from build123d import *

# Parameters (mm, degrees)
SKETCH_1_R          = 25
SKETCH_1_R_2        = 15
EXTRUDE_START       = -20
SKETCH_3_R          = 36
SKETCH_3_R_2        = 25
EXTRUDE_2_DEPTH     = 5
SKETCH_4_W          = 10
SKETCH_4_H          = 4
CUT_EXTRUDE_1_REACH = 133.651
SKETCH_5_R          = 25
SKETCH_5_R_2        = 24
CHAMFER_1_SIZE      = 1.648


with BuildPart() as part:
    # По траектории1: sweep along a path in Эскиз2
    with BuildLine(Plane(origin=(0, 0, 0), x_dir=(1, 0, 0), z_dir=(0, 1, 0))) as sweep_1_path:
        Line((0, 0), (0, -62.679491924))
        ThreePointArc((0, -62.679491924), (-4.019237886, -77.679491924), (-15, -88.660254038))
        Line((-15, -88.660254038), (-51.961524227, -110))
    # Эскиз1 → По траектории1 (sweep)
    with BuildSketch(Plane.XY):
        Circle(SKETCH_1_R)
        Circle(SKETCH_1_R_2, mode=Mode.SUBTRACT)
    sweep(path=sweep_1_path.line)

    # Эскиз3 → Бобышка-Вытянуть2 (add)
    with BuildSketch(Plane(origin=(0, 0, 0), x_dir=(-1, 0, 0), z_dir=(0, 0, -1)).offset(EXTRUDE_START)):
        Circle(SKETCH_3_R)
        Circle(SKETCH_3_R_2, mode=Mode.SUBTRACT)
    extrude(amount=-EXTRUDE_2_DEPTH)

    # Эскиз4 → Вырез-Повернуть1 (revolve, cut)
    with BuildSketch(Plane(origin=(0, 0, 0), x_dir=(1, 0, 0), z_dir=(0, 1, 0))):
        with Locations((27, -18)):
            Rectangle(SKETCH_4_W, SKETCH_4_H)
    revolve(axis=Axis((0, 0, 0), (0, 0, 1)), mode=Mode.SUBTRACT)

    # Эскиз5 → Вырез-Вытянуть1 (cut, up to next)
    with BuildSketch(Plane(origin=(0, 0, 0), x_dir=(-1, 0, 0), z_dir=(0, 0, -1)), mode=Mode.PRIVATE) as cut_extrude_1_sk1:
        Circle(SKETCH_5_R)
        Circle(SKETCH_5_R_2, mode=Mode.SUBTRACT)
    cut_extrude_1_tool1 = extrude(cut_extrude_1_sk1.sketch, amount=-CUT_EXTRUDE_1_REACH, mode=Mode.PRIVATE) & part.part
    add(cut_extrude_1_tool1.solids().sort_by_distance((24.292893, 0, 0))[0], mode=Mode.SUBTRACT)

    # Фаска1
    chamfer_1_edges = [part.edges().sort_by_distance(p)[0] for p in [
        (24, 0, 0),
    ]]
    chamfer(chamfer_1_edges, length=CHAMFER_1_SIZE)


solid = part.part
Design review of the part built by this model. Coordinates are the model's own, in mm. A direction names the side the tool comes from. Round coordinates to 2 decimals unless told otherwise and drop trailing zeros. Write each loop counter-clockwise with the first axis right and the second up, starting at its lowest first coordinate (ties: lowest second). Pieces come first, ordered by that corner, then holes.
Item 1: For faces 4 (the flat face through (-57.342, 10.761, 100.681)), 5 (the cylindrical face through (23.846, 7.509, 44.104)), 6 (the cylindrical face through (-14.985, 0.66, 31.779)), list the 3-axis set-ups (+Z, -Z, +X, -X, +Y, -Y) from which the entire face can be reached by the end or side of a thin tool; tool diameter is ignored.
Item 2: Wall thickness on L1, parallel to Y at x = 0, z = 20.5; L2, parallel to Z at x = 18, y = -27.5; L3, parallel to Y at x = 0, z = 44: over which ranges is each line inside the solid? List them lowest first.
Item 3: For pin 1 Ø8 at (x, y) = (20, 4.5) entering from +Z; pin 2 Ø10 at (x, z) = (-34, 99) entering from +Y; pin 3 Ø14.5 at (x, y) = (1.5, -5.5) entering from +Z, all flat-tipped, find the tip position at first contact; note any pin that passes through.
Item 4: Draft analysis for pull direction Y (two halves, no side actions). For faces 1 (the cylindrical face through (-39.69, -9.13, 89.17)), 2 (the flat face through (-21.2, -7, 16)), 3 (the cylindrical face through (-21.82, 7.51, 120.13)), state which applies: released by +Y, released by -Y, zero draft, split by the parting line, or undercut.
Item 5: Consider section C-C on x = 27. Give the boundary of the cut face in (y, z).
Item 6: Consider section B-B on z = 37. Give the boundary of the cut face in (x, y), and give its area (3 significant figures).
Check values:
1. face 4: +Z, -X, +Y, -Y
1. face 5: none
1. face 6: -Z
2. L1: y = -36 to -15, 15 to 36
2. L2: z = 20 to 25
2. L3: y = -25 to -15, 15 to 25
3. pin 1: stops at z = 92.2
3. pin 2: stops at y = 25
3. pin 3: stops at z = 111.74
4. face 1: undercut
4. face 2: zero draft
4. face 3: split by the parting line
5. outline: (-23.81, 20) - (23.81, 20) - (23.81, 25) - (-23.81, 25) - close
6. outline: circle Ø50 at (0, 0); hole circle Ø30 at (0, 0)
6. area: 1,260 mm2
